```python
from build123d import *

# Parameters (mm, degrees)
SKETCH1_W           = 15
SKETCH1_H           = 20
BOSS_EXTRUDE1_DEPTH = 1.5
SKETCH2_R           = 1
CUT_EXTRUDE1_DEPTH  = 1.5
CUT_EXTRUDE2_DEPTH  = 1.5
CUT_EXTRUDE3_DEPTH  = 1.5


with BuildPart() as part:
    # Sketch1 → Boss-Extrude1 (new body)
    with BuildSketch(Plane(origin=(0, 0, 0), x_dir=(1, 0, 0), z_dir=(0, 1, 0))):
        with Locations((-8.746418338, 3.724928367)):
            Rectangle(SKETCH1_W, SKETCH1_H)
    extrude(amount=BOSS_EXTRUDE1_DEPTH)

    # Sketch2 → Cut-Extrude1 (cut)
    with BuildSketch(Plane(origin=(0, 1.5, 0), x_dir=(1, 0, 0), z_dir=(0, 1, 0))):
        with Locations((-10.120989787, 3.638381578)):
            Circle(SKETCH2_R)
    extrude(amount=-CUT_EXTRUDE1_DEPTH, mode=Mode.SUBTRACT)

    # Sketch3 → Cut-Extrude2 (cut)
    with BuildSketch(Plane(origin=(0, 1.5, 0), x_dir=(1, 0, 0), z_dir=(0, 1, 0))):
        Polygon((-9.246418338, -6.275071633), (-9.246418338, -7.482454252), (1.99298081, -6.056034197), (1.99298081, 15.151348422), (-9.246418338, 13.724928367), (-9.246418338, 6.224928381), (-1.346418338, 6.224928381), (-1.346418338, 1.224928353), (-9.246418338, 1.224928353), align=None)
    extrude(amount=-CUT_EXTRUDE2_DEPTH, mode=Mode.SUBTRACT)

    # Sketch4 → Cut-Extrude3 (cut)
    with BuildSketch(Plane(origin=(0, 1.5, 0), x_dir=(1, 0, 0), z_dir=(0, 1, 0))):
        with BuildLine():
            Line((-6.136798849, 4.138381578), (-0.966349773, 4.138381578))
            Line((-0.966349773, 4.138381578), (-0.966349773, 3.138381578))
            Line((-0.966349773, 3.138381578), (-6.136798849, 3.138381578))
            ThreePointArc((-6.136798849, 3.138381578), (-6.636798849, 3.638381578), (-6.136798849, 4.138381578))
        make_face()
    extrude(amount=-CUT_EXTRUDE3_DEPTH, mode=Mode.SUBTRACT)


solid = part.part
```
For this review, take the finished solid that the model builds, in its own axes (mm). A direction names the side the tool comes from. Round coordinates to 2 decimals unless told otherwise and drop trailing zeros. Loops run counter-clockwise (first coordinate to the right, second up) from the corner with the lowest first, then second, coordinate; pieces in that order, holes last.
(1) We need section D-D (x = -8.75). Give the boundary of the cut face in (y, z).
Returned:
outline: (0, -6.22) - (1.5, -6.22) - (1.5, -1.22) - (0, -1.22) - close
(2) Tool access review of faces 4 (the flat face through (-5, 1, -6.225)), 5 (the flat face through (-1.346, 1, -2)), 6 (the flat face through (-9.246, 1, 2)), 7 (the flat face through (-4, 1, -4.138)): name each direction out of +Z, -Z, +X, -X, +Y, -Y from which nothing blocks a thin tool from reaching the whole face with its end or side.
Returned:
face 4: -Z, +X, +Y, -Y
face 5: +Z, -Z, +X, +Y, -Y
face 6: +Z, +X, +Y, -Y
face 7: +X, +Y, -Y
(3) Mouldability with a two-part tool opening along Z and no side actions: class faces 1 (the cylindrical face through (-6.637, 0.76, -3.627)), 2 (the flat face through (-5, 1, -1.225)), 3 (the flat face through (-9.246, 1, -10)) as released by +Z, released by -Z, zero draft, split by the parting line, or undercut.
Returned:
face 1: undercut
face 2: released by +Z
face 3: zero draft
(4) Wall thickness on line 1 along Z through (x, y) = (-4.75, 0.5); line 2 along X through (y, z) = (1.4, 3.5); line 3 along Z through (x, y) = (-7.5, 1.25): over which ranges is each line inside the solid? List them lowest first.
Returned:
line 1: z = -6.22 to -4.14, -3.14 to -1.22
line 2: x = -16.25 to -9.25
line 3: z = -6.22 to -1.22
(5) Clearance check with a flat-ended pin moving along its axis: P1, Ø0.8, axis at x = -4, y = 1, coming from the -Z side. State where the tip first meets the part, or that it passes through.
Returned:
P1: stops at z = -6.22
(6) We need section C-C (z = 1.25). Give the boundary of the cut face in (x, y).
Returned:
outline: (-16.25, 0) - (-9.25, 0) - (-9.25, 1.5) - (-16.25, 1.5) - close
(7) We need section A-A (x = -5). Give the boundary of the cut face in (y, z), plus the area to 3 significant figures.
Returned:
outline: (0, -6.22) - (1.5, -6.22) - (1.5, -4.14) - (0, -4.14) - close; (0, -3.14) - (1.5, -3.14) - (1.5, -1.22) - (0, -1.22) - close
area: 6.00 mm2
(8) We need section B-B (y = 0.7). Give the boundary of the cut face in (x, z), plus the area to 3 significant figures.
Returned:
outline: (-16.25, -13.72) - (-9.25, -13.72) - (-9.25, -6.22) - (-1.35, -6.22) - (-1.35, -4.14) - (-6.14, -4.14) arc R0.5 cw to (-6.14, -3.14) - (-1.35, -3.14) - (-1.35, -1.22) - (-9.25, -1.22) - (-9.25, 6.28) - (-16.25, 6.28) - close; hole circle Ø2 at (-10.12, -3.64)
area: 171 mm2
